```python
from build123d import *

# Parameters (mm, degrees)
SKETCH1_W                = 30
SKETCH1_H                = 30
BOSS_EXTRUDE1_DEPTH      = 180
BOSS_EXTRUDE2_DEPTH      = 30
BOSS_EXTRUDE2_DEPTH_BACK = 30
SKETCH2_R                = 15
SKETCH2_R_2              = 12


with BuildPart() as part:
    # Sketch1 → Boss-Extrude1 (new body)
    with BuildSketch(Plane(origin=(0, 0, 0), x_dir=(1, 0, 0), z_dir=(0, 1, 0))):
        Rectangle(SKETCH1_W, SKETCH1_H)
    extrude(amount=BOSS_EXTRUDE1_DEPTH)

    # Sketch2 → Boss-Extrude2 (add, two sides: drawn at the far end of the back side and taken through both)
    with BuildSketch(Plane.XY.offset(-BOSS_EXTRUDE2_DEPTH_BACK)):
        Circle(SKETCH2_R)
        with Locations((0, 180)):
            Circle(SKETCH2_R_2)
    extrude(amount=BOSS_EXTRUDE2_DEPTH + BOSS_EXTRUDE2_DEPTH_BACK)


solid = part.part
```
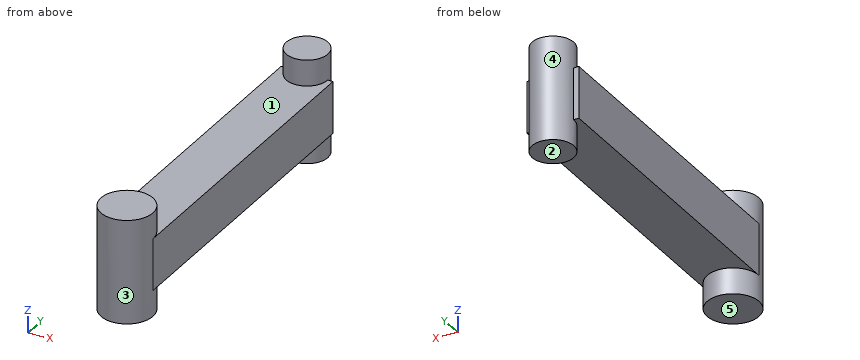
Model file for the job. Use its own axes, mm. Face numbers are marked on the shaded views. A direction names the side the tool comes from. Give positions to 0.01 mm unless a question says otherwise; leave off trailing zeros. Loops run counter-clockwise (first coordinate to the right, second up) from the corner with the lowest first, then second, coordinate; pieces in that order, holes last. Notation, with made-up numbers: M -1.5,35 L 48.5,35 A28 ccw 48.5,57 Z; hole C 37,-15 d11. An arc over 180 degrees is marked long. Use one line per item in the form item = value.
Item 1: Slice it at D-D on y = 160.5. List the corners of the cut face in (x, z).
Filled in:
outline = M -15,-15 L 15,-15 L 15,15 L -15,15 Z
Item 2: Flat gauge pins, fed straight in: pin 1 Ø9 at (x, y) = (-2, 57) entering from +Z; pin 2 Ø1.5 at (x, z) = (-14, -1.5) entering from +Y; pin 3 Ø2 at (x, z) = (-7.5, -9) entering from -Y. Where does each tip first touch, or does it go through?
Filled in:
pin_1 = 15
pin_2 = 180
pin_3 = -13.52
Item 3: Two-plate mould, pull along Y, no slides. Class the marked faces 1, 2 and 3: released by +Y, released by -Y, zero draft, split by the parting line, or undercut.
Filled in:
face_1 = undercut
face_2 = zero draft
face_3 = undercut
Item 4: Which spindle directions (+Z, -Z, +X, -X, +Y, -Y) get a long thin tool onto all of the face, cutting with end or side? Do the marked faces 4 and 5. Say none if no direction does.
Filled in:
face_4 = none
face_5 = -Z, +X, -X, +Y, -Y
Item 5: Slice it at C-C on z = 22. List the corners of the cut face in (x, y), and give its area (3 significant figures).
Filled in:
outline = C 0,0 d30; C 0,180 d24
area = 1,160 mm^2
Item 6: Slice it at A-A on x = 0. List the corners of the cut face in (y, z), and give its area (3 significant figures).
Filled in:
outline = M -15,-30 L 15,-30 L 15,-15 L 168,-15 L 168,-30 L 192,-30 L 192,30 L 168,30 L 168,15 L 15,15 L 15,30 L -15,30 Z
area = 7,830 mm^2
Item 7: Slice it at B-B on z = -7.5. List the corners of the cut face in (x, y), and give its area (3 significant figures).
Filled in:
outline = M -15,0 A15 ccw 15,0 L 15,180 L 12,180 A12 ccw -12,180 L -15,180 Z
area = 5,980 mm^2
Item 8: Drill centre lines: L1, parallel to Z at x = -10.75, y = 108.5; L2, parallel to Y at x = 2.25, z = -27; L3, parallel to Y at x = -3.75, z = 24. Where is each one in solid material? Low to high.
Filled in:
L1 = -15 to 15
L2 = -14.83 to 14.83, 168.21 to 191.79
L3 = -14.52 to 14.52, 168.6 to 191.4
